For this review, take the finished solid that the model builds, in its own axes (mm). Round coordinates to 2 decimals unless told otherwise and drop trailing zeros. Order: outer loops, then holes, each group sorted by start corner. A loop starts at its lowest first (then second) coordinate and runs counter-clockwise, first axis right, second up. Notation, with made-up numbers: (87.25, -5) -> (145.25, -5) arc R31 ccw to (145.25, 22) -> close; hole circle Ø11 at (58, -34.75). An arc over 180 degrees is marked (long way). Put each result on its own line as item: value. Start each with the question number.
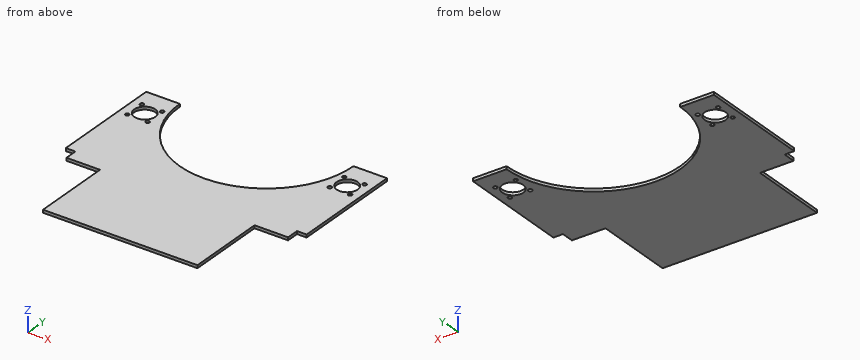
```python
from build123d import *

# Parameters (mm, degrees)
ESQUISSE1_R      = 11
ESQUISSE1_R_2    = 2
EXTRUSION1_DEPTH = 3


with BuildPart() as part:
    # Esquisse1 → Extrusion1 (new body)
    with BuildSketch(Plane.XY):
        with BuildLine():
            Line((125.5, 0), (125.5, -117))
            Line((125.5, -117), (115.5, -117))
            Line((115.5, -117), (115.5, -130))
            Line((115.5, -130), (80.5, -130))
            Line((80.5, -130), (80.5, -213))
            Line((80.5, -213), (-80.5, -213))
            Line((-80.5, -213), (-80.5, -130))
            Line((-80.5, -130), (-115.5, -130))
            Line((-115.5, -130), (-115.5, -117))
            Line((-115.5, -117), (-125.5, -117))
            Line((-125.5, -117), (-125.5, 0))
            Line((-125.5, 0), (-90.5, 0))
            ThreePointArc((-90.5, 0), (0, -90.5), (90.5, 0))
            Line((90.5, 0), (125.5, 0))
        make_face()
        with Locations((-105.5, -30)):
            Circle(ESQUISSE1_R, mode=Mode.SUBTRACT)
        with Locations((116.106601718, -19.393398282)):
            Circle(ESQUISSE1_R_2, mode=Mode.SUBTRACT)
        with Locations((94.893398282, -40.606601718)):
            Circle(ESQUISSE1_R_2, mode=Mode.SUBTRACT)
        with Locations((-94.893398282, -19.393398282)):
            Circle(ESQUISSE1_R_2, mode=Mode.SUBTRACT)
        with Locations((-116.106601718, -40.606601718)):
            Circle(ESQUISSE1_R_2, mode=Mode.SUBTRACT)
        with Locations((-94.893398282, -40.606601718)):
            Circle(ESQUISSE1_R_2, mode=Mode.SUBTRACT)
        with Locations((116.106601718, -40.606601718)):
            Circle(ESQUISSE1_R_2, mode=Mode.SUBTRACT)
        with Locations((94.893398282, -19.393398282)):
            Circle(ESQUISSE1_R_2, mode=Mode.SUBTRACT)
        with Locations((105.5, -30)):
            Circle(ESQUISSE1_R, mode=Mode.SUBTRACT)
        with Locations((-116.106601718, -19.393398282)):
            Circle(ESQUISSE1_R_2, mode=Mode.SUBTRACT)
    extrude(amount=EXTRUSION1_DEPTH)


solid = part.part
```
Item 1: For L1, parallel to Y at x = 103, z = 2; L2, parallel to X at y = -14, z = 1.75; L3, parallel to Y at x = -105.5, z = 1.3, list the stretches that pass through material, from the lowest coordinate up.
Item 2: Insertion check: pin 1 Ø0.9 at (x, z) = (122.5, 1) entering from -Y; pin 2 Ø1.5 at (y, z) = (-125, 1.5) entering from -X; pin 3 Ø0.9 at (y, z) = (-153, 1.5) entering from +X. Each pin has a flat end and moves straight along its axis. Give the tip position at first contact, or say it passes through.
Item 3: Consider section D-D, the plane y = -134.5. Write out the cut boundary in (x, z).
Item 4: Consider section B-B, the plane y = -30. Write out the cut boundary in (x, z), plus the area to 3 significant figures.
Item 5: Consider section A-A, the plane x = -105.5. Write out the cut boundary in (y, z), plus the area to 3 significant figures.
Item 6: Consider section C-C, the plane z = 0.95. Count the separate pieces of the cut face and the enclosed holes in it, plus the area to 3 significant figures.
Evaluation:
1. L1: y = -130 to -40.71, -19.29 to 0
1. L2: x = -125.5 to -89.41, 89.41 to 125.5
1. L3: y = -130 to -41, -19 to 0
2. pin 1: stops at y = -117
2. pin 2: stops at x = -115.5
2. pin 3: stops at x = 80.5
3. outline: (-80.5, 0) -> (80.5, 0) -> (80.5, 3) -> (-80.5, 3) -> close
4. outline: (-125.5, 0) -> (-116.5, 0) -> (-116.5, 3) -> (-125.5, 3) -> close; (-94.5, 0) -> (-85.38, 0) -> (-85.38, 3) -> (-94.5, 3) -> close; (85.38, 0) -> (94.5, 0) -> (94.5, 3) -> (85.38, 3) -> close; (116.5, 0) -> (125.5, 0) -> (125.5, 3) -> (116.5, 3) -> close
4. area: 109 mm^2
5. outline: (-130, 0) -> (-41, 0) -> (-41, 3) -> (-130, 3) -> close; (-19, 0) -> (0, 0) -> (0, 3) -> (-19, 3) -> close
5. area: 324 mm^2
6. separate pieces: 1
6. enclosed holes: 10
6. area: 32,000 mm^2
